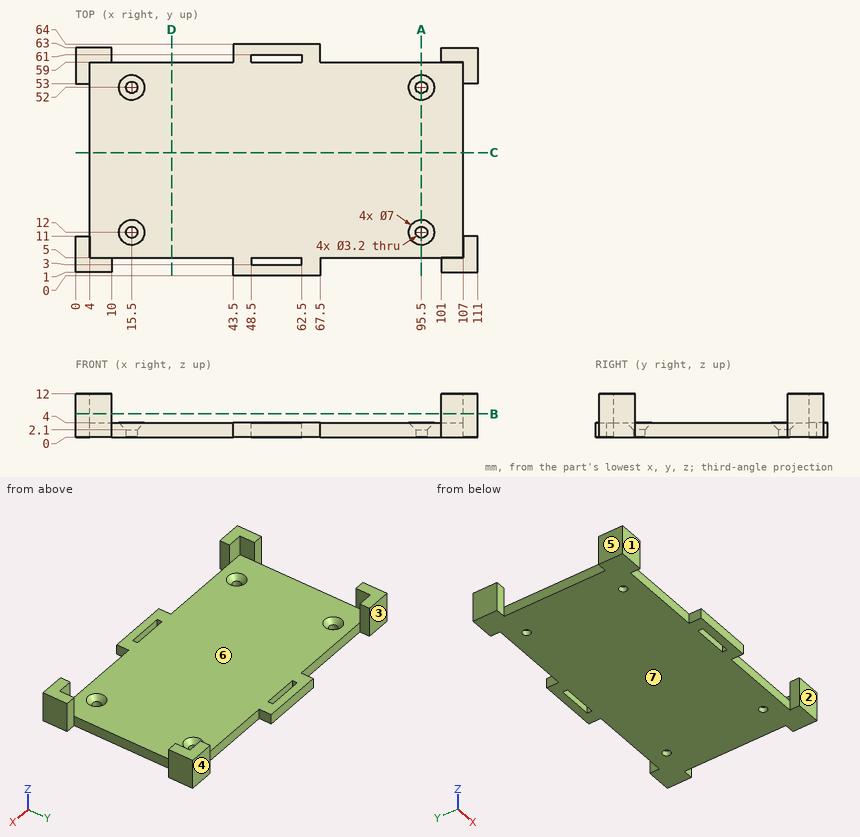
For this review, use the dimensioned drawing (mm, ordinates from the lowest corner) and the shaded views. A direction names the side the tool comes from. Coordinates: 2 decimals unless noted, no trailing zeros. Loops run counter-clockwise (first coordinate to the right, second up) from the corner with the lowest first, then second, coordinate; pieces in that order, holes last. Notation, with made-up numbers: M 10.5,41 L 59.5,41 A22 ccw 59.5,63 Z; hole C 18.5,18 d11. An arc over 180 degrees is marked long. Answer as CSV lines item,"result".
Item 1: For P1, Ø2, axis at x = 55.5, y = 49, coming from the -Z side; P2, Ø3, axis at x = 102.5, z = 8.5, coming from the +Y side; P3, Ø2, axis at x = 25.5, z = 2, coming from the -Y side; P4, Ø3, axis at x = 7.5, z = 8.5, coming from the -Y side, all flat-tipped, find the tip position at first contact; note any pin that passes through.
Answer list:
P1,"z = 0"
P2,"y = 63"
P3,"y = 5"
P4,"y = 1"
Item 2: Add section C-C on y = 34. State the section outline as (x, z) points, plus the area to 3 significant figures.
Answer list:
outline,"M 4,0 L 107,0 L 107,4 L 4,4 Z"
area,"412 mm²"
Item 3: Add section A-A on x = 95.5. State the section outline as (y, z) points, plus the area to 3 significant figures.
Answer list:
outline,"M 5,0 L 10.4,0 L 10.4,2.1 L 8.5,4 L 5,4 Z; M 13.6,0 L 50.4,0 L 50.4,2.1 L 48.5,4 L 15.5,4 L 13.6,2.1 Z; M 53.6,0 L 59,0 L 59,4 L 55.5,4 L 53.6,2.1 Z"
area,"183 mm²"
Item 4: Add section D-D on x = 26.5. State the section outline as (y, z) points.
Answer list:
outline,"M 5,0 L 59,0 L 59,4 L 5,4 Z"
Item 5: For probe 1 along Y at (x, z) = (15.5, 1.65); probe 2 along X at (y, z) = (52, 0.55); probe 3 along X at (y, z) = (4, 3.75), list the stretches that pass through material, from the lowest coordinate up.
Answer list:
probe 1,"5 to 10.4, 13.6 to 50.4, 53.6 to 59"
probe 2,"4 to 13.9, 17.1 to 93.9, 97.1 to 107"
probe 3,"0 to 10, 43.5 to 48.5, 62.5 to 67.5, 101 to 111"
Item 6: The part is to be moulded in two halves that separate along X. For the marked faces 5, 6 and 7, say which applies: pulls with the +X half, pulls with the -X half, needs draft (parallel to the pull), parting line crosses it, or undercut.
Answer list:
face 5,"pulls with the -X half"
face 6,"undercut"
face 7,"needs draft"
Item 7: Add section B-B on z = 6.5. State the section outline as (x, y) points.
Answer list:
outline,"M 0,1 L 10,1 L 10,5 L 4,5 L 4,11 L 0,11 Z; M 0,53 L 4,53 L 4,59 L 10,59 L 10,63 L 0,63 Z; M 101,1 L 111,1 L 111,11 L 107,11 L 107,5 L 101,5 Z; M 101,59 L 107,59 L 107,53 L 111,53 L 111,63 L 101,63 Z"
Item 8: Machinability: for the marked faces 1, 2, 3 and 4, which of the approach directions +Z, -Z, +X, -X, +Y, -Y give a long, thin tool a straight path to every point of the face, cutting with its end or side? Answer none if there is none.
Answer list:
face 1,"+Z, -Z, -X, -Y"
face 2,"+Z, -Z, +X, -Y"
face 3,"+Z, -Z, -X, +Y"
face 4,"+Z, -Z, +X, +Y"
